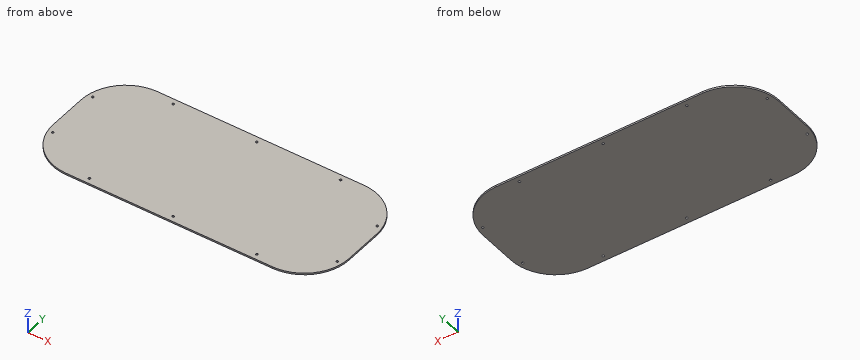
from build123d import *

# Parameters (mm, degrees)
SKETCH_1_W          = 530
SKETCH_1_H          = 230
EXTRUDE_1_DEPTH     = 3
FILLET_1_R          = 80
SKETCH_2_R          = 2
CUT_EXTRUDE_1_DEPTH = 10


with BuildPart() as part:
    # 草图1 → 凸台-拉伸1 (new body)
    with BuildSketch(Plane.XY):
        Rectangle(SKETCH_1_W, SKETCH_1_H)
    extrude(amount=EXTRUDE_1_DEPTH)

    # 圆角1
    fillet_1_edges = [part.edges().sort_by_distance(p)[0] for p in [
        (265, -115, 1.5),
        (-265, -115, 1.5),
        (-265, 115, 1.5),
        (265, 115, 1.5),
    ]]
    fillet(fillet_1_edges, radius=FILLET_1_R)

    # 草图2 → 切除-拉伸1 (cut)
    with BuildSketch(Plane.XY.offset(3)):
        with Locations((-255, -50)):
            Circle(SKETCH_2_R)
        with Locations((-255, 50)):
            Circle(SKETCH_2_R)
        with Locations((-150, -105)):
            Circle(SKETCH_2_R)
        with Locations((0, -105)):
            Circle(SKETCH_2_R)
        with Locations((150, -105)):
            Circle(SKETCH_2_R)
        with Locations((255, -50)):
            Circle(SKETCH_2_R)
        with Locations((255, 50)):
            Circle(SKETCH_2_R)
        with Locations((150, 105)):
            Circle(SKETCH_2_R)
        with Locations((0, 105)):
            Circle(SKETCH_2_R)
        with Locations((-150, 105)):
            Circle(SKETCH_2_R)
    extrude(amount=-CUT_EXTRUDE_1_DEPTH, mode=Mode.SUBTRACT)


solid = part.part
Verification items for the finished model (mm, model axes). Give positions to 0.01 mm unless a question says otherwise; leave off trailing zeros. Loops run counter-clockwise (first coordinate to the right, second up) from the corner with the lowest first, then second, coordinate; pieces in that order, holes last.
1. Cross-section at C-C on y = -70.5. Record the cut outline in (x, z).
Derived:
outline: (-256.69, 0) - (256.69, 0) - (256.69, 3) - (-256.69, 3) - close
2. Cross-section at A-A on z = 1.15. Count the separate pieces of the cut face and the enclosed holes in it, and give its area (3 significant figures).
Derived:
separate pieces: 1
enclosed holes: 10
area: 116,000 mm2
3. Material ranges on probe 1 along Y at (x, z) = (-150, 2.3); probe 2 along Y at (x, z) = (-255, 1.8); probe 3 along X at (y, z) = (-80, 0.4), recorded low to high.
Derived:
probe 1: y = -115 to -107, -103 to 103, 107 to 115
probe 2: y = -73.73 to -52, -48 to 48, 52 to 73.73
probe 3: x = -251.14 to 251.14
4. Cross-section at B-B on x = 231. Record the cut outline in (y, z), and give its area (3 significant figures).
Derived:
outline: (-100.45, 0) - (100.45, 0) - (100.45, 3) - (-100.45, 3) - close
area: 603 mm2
5. Go/stop test with flat-tipped pins: P1, Ø4.5, axis at x = 0, y = -105, coming from the -Z side; P2, Ø1, axis at y = -85.5, z = 1.5, coming from the +X side. Record where each tip stops, or that it passes through.
Derived:
P1: stops at z = 0
P2: stops at x = 247.45
